Geometry check sheet. Reference: the model listing, model coordinates, mm. Face numbers are marked on the shaded views. A direction names the side the tool comes from. Coordinates: 2 decimals unless noted, no trailing zeros. Write each loop counter-clockwise with the first axis right and the second up, starting at its lowest first coordinate (ties: lowest second). Pieces come first, ordered by that corner, then holes.
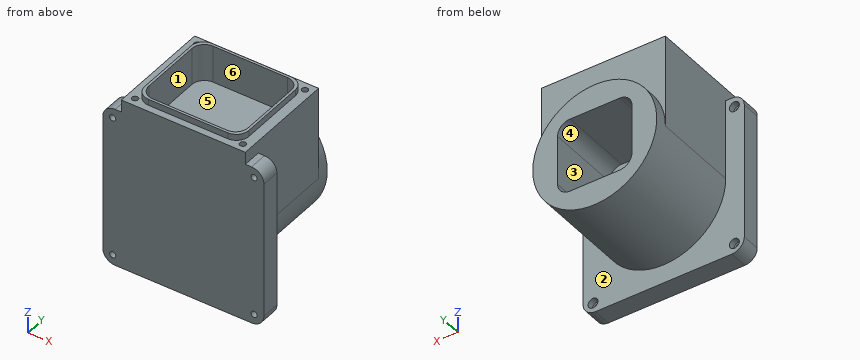
from build123d import *

# Parameters (mm, degrees)
SKETCH1_W           = 130
SKETCH1_H           = 130
BOSS_EXTRUDE1_DEPTH = 15
SKETCH2_R           = 50
BOSS_EXTRUDE2_DEPTH = 80
SKETCH3_W           = 75
SKETCH3_H           = 85
BOSS_EXTRUDE3_DEPTH = 50
CUT_EXTRUDE2_DEPTH  = 60
CUT_EXTRUDE4_DEPTH  = 25
SKETCH6_R           = 2.5
CUT_EXTRUDE5_DEPTH  = 35
FILLET1_R           = 10
BOSS_EXTRUDE5_DEPTH = 5
SKETCH8_R           = 2.5
CUT_EXTRUDE6_DEPTH  = 16
SKETCH9_R           = 4
CUT_EXTRUDE7_DEPTH  = 5


with BuildPart() as part:
    # Sketch1 → Boss-Extrude1 (new body)
    with BuildSketch(Plane(origin=(0, 0, 0), x_dir=(1, 0, 0), z_dir=(0, 1, 0))):
        Rectangle(SKETCH1_W, SKETCH1_H)
    extrude(amount=BOSS_EXTRUDE1_DEPTH)

    # Sketch2 → Boss-Extrude2 (add)
    with BuildSketch(Plane(origin=(0, 15, 0), x_dir=(1, 0, 0), z_dir=(0, 1, 0))):
        Circle(SKETCH2_R)
    extrude(amount=BOSS_EXTRUDE2_DEPTH)

    # Sketch3 → Boss-Extrude3 (add, symmetric)
    with BuildSketch(Plane(origin=(0, 0, 0), x_dir=(0, 0, -1), z_dir=(1, 0, 0))):
        with Locations((-37.5, 42.5)):
            Rectangle(SKETCH3_W, SKETCH3_H)
    extrude(amount=BOSS_EXTRUDE3_DEPTH, both=True)

    # Sketch4 → Cut-Extrude2 (cut)
    with BuildSketch(Plane(origin=(0, 95, 0), x_dir=(1, 0, 0), z_dir=(0, 1, 0))):
        with BuildLine():
            Line((-20, 30), (20, 30))
            ThreePointArc((20, 30), (27.071067812, 27.071067812), (30, 20))
            Line((30, 20), (30, -20))
            ThreePointArc((30, -20), (27.071067812, -27.071067812), (20, -30))
            Line((20, -30), (-20, -30))
            ThreePointArc((-20, -30), (-27.071067812, -27.071067812), (-30, -20))
            Line((-30, -20), (-30, 20))
            ThreePointArc((-30, 20), (-27.071067812, 27.071067812), (-20, 30))
        make_face()
    extrude(amount=-CUT_EXTRUDE2_DEPTH, mode=Mode.SUBTRACT)

    # Sketch5 → Cut-Extrude4 (cut)
    with BuildSketch(Plane.XY.offset(75)):
        with BuildLine():
            Line((-30, 77.5), (30, 77.5))
            ThreePointArc((30, 77.5), (37.071067812, 74.571067812), (40, 67.5))
            Line((40, 67.5), (40, 17.5))
            ThreePointArc((40, 17.5), (37.071067812, 10.428932188), (30, 7.5))
            Line((30, 7.5), (-30, 7.5))
            ThreePointArc((-30, 7.5), (-37.071067812, 10.428932188), (-40, 17.5))
            Line((-40, 17.5), (-40, 67.5))
            ThreePointArc((-40, 67.5), (-37.071067812, 74.571067812), (-30, 77.5))
        make_face()
    extrude(amount=-CUT_EXTRUDE4_DEPTH, mode=Mode.SUBTRACT)

    # Sketch6 → Cut-Extrude5 (cut)
    with BuildSketch(Plane.XY.offset(75)):
        with Locations((-43.5, 78.5)):
            Circle(SKETCH6_R)
        with Locations((43.5, 78.5)):
            Circle(SKETCH6_R)
        with Locations((43.5, 6.5)):
            Circle(SKETCH6_R)
        with Locations((-43.5, 6.5)):
            Circle(SKETCH6_R)
    extrude(amount=-CUT_EXTRUDE5_DEPTH, mode=Mode.SUBTRACT)

    # Fillet1
    fillet1_edges = [part.edges().sort_by_distance(p)[0] for p in [
        (65, 7.5, 65),
        (-65, 7.5, 65),
        (-65, 7.5, -65),
        (65, 7.5, -65),
    ]]
    fillet(fillet1_edges, radius=FILLET1_R)

    # Sketch7 → Boss-Extrude5 (add)
    with BuildSketch(Plane.XY.offset(75)):
        with BuildLine():
            Line((-32, 79.5), (32, 79.5))
            ThreePointArc((32, 79.5), (39.071067812, 76.571067812), (42, 69.5))
            Line((42, 69.5), (42, 15.5))
            ThreePointArc((42, 15.5), (39.071067812, 8.428932188), (32, 5.5))
            Line((32, 5.5), (-32, 5.5))
            ThreePointArc((-32, 5.5), (-39.071067812, 8.428932188), (-42, 15.5))
            Line((-42, 15.5), (-42, 69.5))
            ThreePointArc((-42, 69.5), (-39.071067812, 76.571067812), (-32, 79.5))
        make_face()
        with BuildLine():
            Line((-30, 77.5), (30, 77.5))
            ThreePointArc((30, 77.5), (37.071067812, 74.571067812), (40, 67.5))
            Line((40, 67.5), (40, 17.5))
            ThreePointArc((40, 17.5), (37.071067812, 10.428932188), (30, 7.5))
            Line((30, 7.5), (-30, 7.5))
            ThreePointArc((-30, 7.5), (-37.071067812, 10.428932188), (-40, 17.5))
            Line((-40, 17.5), (-40, 67.5))
            ThreePointArc((-40, 67.5), (-37.071067812, 74.571067812), (-30, 77.5))
        make_face(mode=Mode.SUBTRACT)
    extrude(amount=BOSS_EXTRUDE5_DEPTH)

    # Sketch8 → Cut-Extrude6 (cut, through all)
    with BuildSketch(Plane(origin=(0, 15, 0), x_dir=(1, 0, 0), z_dir=(0, 1, 0))):
        with Locations((-57, 57)):
            Circle(SKETCH8_R)
        with Locations((-57, -57)):
            Circle(SKETCH8_R)
        with Locations((57, -57)):
            Circle(SKETCH8_R)
        with Locations((57, 57)):
            Circle(SKETCH8_R)
    extrude(amount=-CUT_EXTRUDE6_DEPTH, mode=Mode.SUBTRACT)

    # Sketch9 → Cut-Extrude7 (cut)
    with BuildSketch(Plane(origin=(0, 15, 0), x_dir=(1, 0, 0), z_dir=(0, 1, 0))):
        with Locations((-57, 57)):
            Circle(SKETCH9_R)
        with Locations((57, 57)):
            Circle(SKETCH9_R)
        with Locations((-57, -57)):
            Circle(SKETCH9_R)
        with Locations((57, -57)):
            Circle(SKETCH9_R)
    extrude(amount=-CUT_EXTRUDE7_DEPTH, mode=Mode.SUBTRACT)


solid = part.part
1. Sectioned sample at B-B, the plane z = -57. Record the boundary of the cut face in (x, y), and give its area (3 significant figures).
Computed values:
outline: (-64.8, 0) - (-59.5, 0) - (-59.5, 10) - (-61, 10) - (-61, 15) - (-64.8, 15) - close; (-54.5, 0) - (54.5, 0) - (54.5, 10) - (53, 10) - (53, 15) - (-53, 15) - (-53, 10) - (-54.5, 10) - close; (59.5, 0) - (64.8, 0) - (64.8, 15) - (61, 15) - (61, 10) - (59.5, 10) - close
area: 1,760 mm2
2. Sectioned sample at A-A, the plane x = 0. Record the boundary of the cut face in (y, z).
Computed values:
outline: (0, -65) - (15, -65) - (15, -50) - (95, -50) - (95, -30) - (35, -30) - (35, 30) - (95, 30) - (95, 50) - (85, 50) - (85, 75) - (79.5, 75) - (79.5, 80) - (77.5, 80) - (77.5, 50) - (7.5, 50) - (7.5, 80) - (5.5, 80) - (5.5, 75) - (0, 75) - close
3. Access from +Z, -Z, +X, -X, +Y, -Y to the whole of each face (thin tool, end or side, straight path). Record for the marked faces 1, 2 and 3.
Computed values:
face 1: +Z
face 2: -Z, +Y
face 3: +Y
4. Thickness scan on line 1 along Y through (x, z) = (43.5, 56.5); line 2 along X through (y, z) = (73, 13.5); line 3 along Z through (x, y) = (-1, 83.5). Record the ranges inside material, lowest first.
Computed values:
line 1: y = 0 to 4, 9 to 76, 81 to 85
line 2: x = -50 to -30, 30 to 50
line 3: z = -49.99 to -30, 30 to 75
5. Draft check along Z on the marked faces 4, 5 and 6. Enter one of: released by +Z, released by -Z, zero draft, split by the parting line, or undercut.
Computed values:
face 4: undercut
face 5: released by +Z
face 6: zero draft
6. Sectioned sample at C-C, the plane y = 39.5. Record the boundary of the cut face in (x, z), and give its area (3 significant figures).
Computed values:
outline: (-50, 0) arc R50 ccw to (50, 0) - (50, 75) - (42, 75) - (42, 80) - (40, 80) - (40, 50) - (-40, 50) - (-40, 80) - (-42, 80) - (-42, 75) - (-50, 75) - close; hole (-30, -20) arc R10 ccw to (-20, -30) - (20, -30) arc R10 ccw to (30, -20) - (30, 20) arc R10 ccw to (20, 30) - (-20, 30) arc R10 ccw to (-30, 20) - close
area: 5,930 mm2
7. Gauge pin test, flat ends, axial feed: pin 1 Ø10 at (x, y) = (30.5, 42.5) entering from +Z; pin 2 Ø2.5 at (x, z) = (-12, 78.5) entering from -Y; pin 3 Ø3 at (x, z) = (10.5, 14) entering from +Y; pin 4 Ø4 at (x, z) = (-57, -57) entering from -Y. Record the tip position at first contact, or that the pin passes through.
Computed values:
pin 1: stops at z = 50
pin 2: stops at y = 5.5
pin 3: stops at y = 35
pin 4: passes through
8. Sectioned sample at D-D, the plane x = 57. Record the boundary of the cut face in (y, z).
Computed values:
outline: (0, -64.8) - (15, -64.8) - (15, -61) - (10, -61) - (10, -59.5) - (0, -59.5) - close; (0, -54.5) - (10, -54.5) - (10, -53) - (15, -53) - (15, 53) - (10, 53) - (10, 54.5) - (0, 54.5) - close; (0, 59.5) - (10, 59.5) - (10, 61) - (15, 61) - (15, 64.8) - (0, 64.8) - close
